For this review, take the finished solid that the model builds, in its own axes (mm). A direction names the side the tool comes from. Coordinates: 2 decimals unless noted, no trailing zeros. Loops run counter-clockwise (first coordinate to the right, second up) from the corner with the lowest first, then second, coordinate; pieces in that order, holes last. Notation, with made-up numbers: M 40,77.25 L 54,77.25 A35 ccw 54,116.25 Z; hole C -31,-11.5 d7. An arc over 180 degrees is marked long. Answer as a JSON object with one key per item and string values. Group by question number.
Item 1: Add section A-A (z = -76.5). State the section outline as (x, y) points, then the cut area to 3 significant figures.
Item 2: Wall thickness on L1, parallel to X at y = 0.5, z = -20.5: over which ranges is the line inside the solid? List them lowest first. Write a range as from..to.
Item 3: Mouldability with a two-part tool opening along X and no side actions: class faces 3 (the face through (-0.86, 2.54, -84.1)), 4 (the face through (-82.5, 2, -43)), 5 (the face through (-39, 0, -83)) as +X half, -X half, draft (parallel to the pull), parting line (faces both ways), or undercut.
Item 4: Add section B-B (y = 3.1). State the section outline as (x, z) points, then the cut area to 3 significant figures.
Item 5: Tool access review of faces 1 (the face through (-2.5, 2, -42)), 2 (the face through (0, 2, -43)): name each direction out of +Z, -Z, +X, -X, +Y, -Y from which nothing blocks a thin tool from reaching the whole face with its end or side.
Item 6: Add section C-C (x = -53.5). State the section outline as (y, z) points.
Autodesk Inventor part; units mm, degrees
ref_plane "YZ Plane" through (0, 0, 0) normal (1, 0, 0) x (0, 1, 0)
ref_plane "XZ Plane" through (0, 0, 0) normal (0, 1, 0) x (-1, 0, 0)
ref_plane "XY Plane" through (0, 0, 0) normal (0, 0, 1) x (1, 0, 0)
sketch "スケッチ1" plane through (0, 0, 0) normal (0, 1, 0) x (-1, 0, 0)
  line L0 (0, 0) -> (85, 0)
  line L1 (85, 0) -> (85, -85)
  line L2 (85, -85) -> (0, -85)
  line L3 (0, -85) -> (0, 0)
  line L4 (82.5, -2.5) -> (2.5, -2.5)
  line L5 (2.5, -2.5) -> (2.5, -82.5)
  line L6 (2.5, -82.5) -> (82.5, -82.5)
  line L7 (82.5, -82.5) -> (82.5, -2.5)
  point P0 (42.5, -2.5)
  point P1 (42.5, 0)
  point P2 (82.5, -42.5)
  point P3 (85, -42.5)
  dimension "d0" = 85
  dimension "d1" = 85
  dimension "d2" = 80
  dimension "d3" = 80
extrude "押し出し1" add sketch "スケッチ1" along normal blind 5
fillet "フィレット1" radius 3 4 edges at (0, 2.5, 0) (-85, 2.5, 0) (-85, 2.5, -85) (0, 2.5, -85)
properties part number "こたつの足_試作"
From the geometry:
{
 "1": {"outline": "M -85,0 L -82.5,0 L -82.5,5 L -85,5 Z; M -2.5,0 L 0,0 L 0,5 L -2.5,5 Z", "area": "25.0 mm²"},
 "2": {"L1": "x = -85..-82.5, -2.5..0"},
 "3": {"face 3": "+X half", "face 4": "undercut", "face 5": "draft"},
 "4": {"outline": "M -85,-82 A3 ccw -82,-85 L -3,-85 A3 ccw 0,-82 L 0,-3 A3 ccw -3,0 L -82,0 A3 ccw -85,-3 Z; hole M -82.5,-82.5 L -2.5,-82.5 L -2.5,-2.5 L -82.5,-2.5 Z", "area": "817 mm²"},
 "5": {"face 1": "+Y, -Y", "face 2": "+Z, -Z, +X, +Y, -Y"},
 "6": {"outline": "M 0,-85 L 5,-85 L 5,-82.5 L 0,-82.5 Z; M 0,-2.5 L 5,-2.5 L 5,0 L 0,0 Z"}
}
